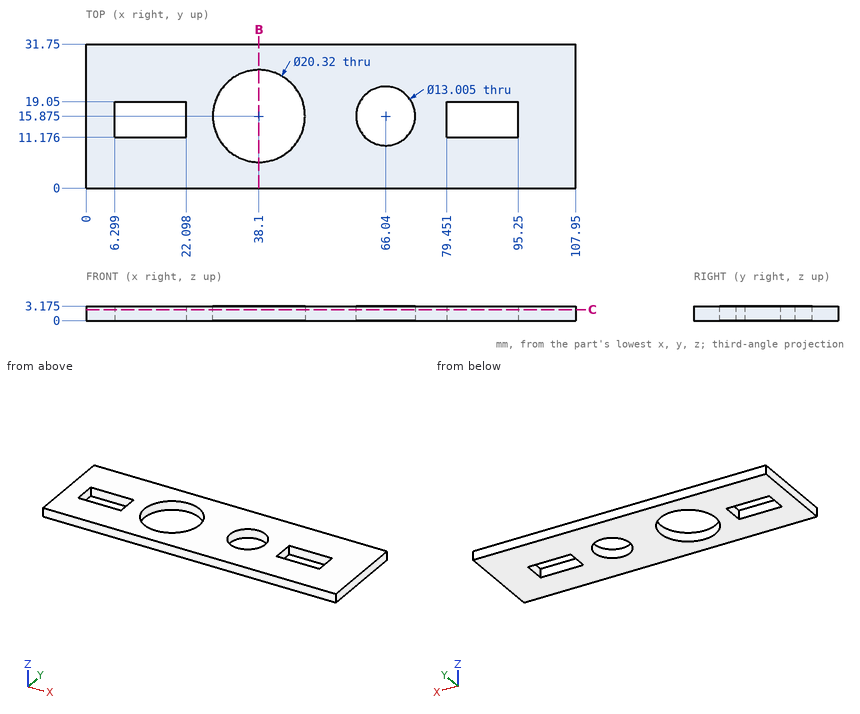
Geometry: see drawing. Coordinates: mm, zero at the bounding-box minimum. Round coordinates to 2 decimals unless told otherwise and drop trailing zeros. Loops run counter-clockwise (first coordinate to the right, second up) from the corner with the lowest first, then second, coordinate; pieces in that order, holes last. Notation, with made-up numbers: (46, 74.25) -> (95, 74.25) arc R29 cw to (95, 105.25) -> close; hole circle Ø3 at (68.25, 1.25). An arc over 180 degrees is marked (long way). Write each question's results on one line, items separated by ' | '.
1. Ray query, line 1 (Y direction, x = 81.5, z = 0.55); line 2 (Y direction, x = 38.1, z = 1.65) (3 decimals); line 3 (X direction, y = 12, z = 0.45). Return the intervals inside material, ascending. Write a range as from..to.
Geometry results:
line 1: 0..11.18, 19.05..31.75 | line 2: 0..5.715, 26.035..31.75 | line 3: 0..6.3, 22.1..28.71, 47.49..60.82, 71.26..79.45, 95.25..107.95
2. Section B-B (x = 38.1). Return loops of the section in (y, z) (3 decimals).
Geometry results:
outline: (0, 0) -> (5.715, 0) -> (5.715, 3.175) -> (0, 3.175) -> close; (26.035, 0) -> (31.75, 0) -> (31.75, 3.175) -> (26.035, 3.175) -> close
3. Section C-C (z = 2.4). State how many separate pieces and enclosed holes the cut face has, and give its area (3 significant figures).
Geometry results:
separate pieces: 1 | enclosed holes: 4 | area: 2,720 mm2
4. First-contact query: P1, Ø15, axis at x = 66.04, y = 15.875, coming from the -Z side. Flat tip, straight axial feed; report the tip coordinate or a pass-through.
Geometry results:
P1: z = 0
